Check sheet for the modelled part. Datum: model origin and axes. Units: mm. A direction names the side the tool comes from. Round coordinates to 2 decimals unless told otherwise and drop trailing zeros. Order: outer loops, then holes, each group sorted by start corner. A loop starts at its lowest first (then second) coordinate and runs counter-clockwise, first axis right, second up. Notation, with made-up numbers: (19.25, -35.75) -> (78.25, -35.75) arc R5 cw to (78.25, -31.75) -> close; hole circle Ø10 at (1.25, 87). An arc over 180 degrees is marked (long way). Answer in a Markdown table with one row per item. Add a question column.
1. Depth check by flat-ended pin: P1, Ø1, axis at y = 14, z = 1, coming from the +X side; P2, Ø0.5, axis at x = -56, z = 2, coming from the +Y side; P3, Ø0.6, axis at y = 13.5, z = 1.5, coming from the -X side. Enter the tip coordinate at first touch or a pass-through.
2. Sectioned sample at C-C, the plane x = 51. Record the boundary of the cut face in (y, z), then the cut area to 3 significant figures.
3. Material ranges on L1, parallel to Y at x = 9, z = 1.55; L2, parallel to X at y = 10.5, z = 0.35; L3, parallel to X at y = 9, z = 1.85, recorded low to high. Write a range as from..to.
4. Access from +Z, -Z, +X, -X, +Y, -Y to the whole of each face (thin tool, end or side, straight path). Record for faces 1 (the flat face through (1, 0, 0)), 2 (the flat face through (-55.525, -5, 2)).
5. Draft check along X on faces 3 (the cylindrical face through (4.18, 5.45, 1.52)), 4 (the flat face through (1, 0, 3)), 5 (the cylindrical face through (55.273, 12.743, 1.479)). Enter one of: +X half, -X half, draft (parallel to the pull), parting line (faces both ways), or undercut.
6. Sectioned sample at B-B, the plane y = -2.25. Record the boundary of the cut face in (x, z) (3 decimals), then the cut area to 3 significant figures.
7. Sectioned sample at A-A, the plane z = 1.2. Record the boundary of the cut face in (x, y) (3 decimals).
8. Sectioned sample at D-D, the plane y = 12. Record the boundary of the cut face in (x, z), then the cut area to 3 significant figures.
```python
from build123d import *

# Parameters (mm, degrees)
SKETCH1_R           = 3.8
BOSS_EXTRUDE2_DEPTH = 3
SKETCH2_R           = 4.4
BOSS_EXTRUDE3_DEPTH = 25
CUT_EXTRUDE3_START  = -1
SKETCH10_R          = 4.4
CUT_EXTRUDE3_DEPTH  = 1
CUT_EXTRUDE4_DEPTH  = 50
SKETCH12_R          = 4.55
CUT_EXTRUDE6_DEPTH  = 50
CUT_EXTRUDE7_DEPTH  = 25


with BuildPart() as part:
    # Sketch1 → Boss-Extrude2 (new body)
    with BuildSketch(Plane.XY):
        with BuildLine():
            Line((-48.125, 15.75), (48.125, 15.75))
            ThreePointArc((48.125, 15.75), (55.196067812, 12.821067812), (58.125, 5.75))
            Line((58.125, 5.75), (58.125, -15.75))
            Line((58.125, -15.75), (-58.125, -15.75))
            Line((-58.125, -15.75), (-58.125, 5.75))
            ThreePointArc((-58.125, 5.75), (-55.196067812, 12.821067812), (-48.125, 15.75))
        make_face()
        with Locations((31.875, -2.25)):
            Circle(SKETCH1_R, mode=Mode.SUBTRACT)
        with Locations((-31.875, 0.25)):
            Circle(SKETCH1_R, mode=Mode.SUBTRACT)
    extrude(amount=BOSS_EXTRUDE2_DEPTH)

    # Sketch2 → Boss-Extrude3 (add)
    with BuildSketch(Plane.XY.offset(3)):
        with Locations((8.725, 5.25)):
            Circle(SKETCH2_R)
        with Locations((-10.185, -4.75)):
            Circle(SKETCH2_R)
        with BuildLine():
            Line((55.625, 5.75), (55.625, -15.75))
            Line((55.625, -15.75), (58.125, -15.75))
            Line((58.125, -15.75), (58.125, 5.25))
            Line((58.125, 5.25), (58.125, 5.75))
            ThreePointArc((58.125, 5.75), (55.196067812, 12.821067812), (48.125, 15.75))
            Line((48.125, 15.75), (48.125, 13.25))
            ThreePointArc((48.125, 13.25), (53.428300859, 11.053300859), (55.625, 5.75))
        make_face()
        with BuildLine():
            Line((-58.125, -15.75), (-55.625, -15.75))
            Line((-55.625, -15.75), (-55.625, 5.75))
            ThreePointArc((-55.625, 5.75), (-53.428300859, 11.053300859), (-48.125, 13.25))
            Line((-48.125, 13.25), (-48.125, 15.75))
            ThreePointArc((-48.125, 15.75), (-55.196067812, 12.821067812), (-58.125, 5.75))
            Line((-58.125, 5.75), (-58.125, 5.25))
            Line((-58.125, 5.25), (-58.125, -15.75))
        make_face()
    extrude(amount=BOSS_EXTRUDE3_DEPTH)

    # Sketch10 → Cut-Extrude3 (cut)
    with BuildSketch(Plane.XY.offset(28).offset(CUT_EXTRUDE3_START)):
        with Locations((8.725, 5.25)):
            Circle(SKETCH10_R)
        with Locations((-10.185, -4.75)):
            Circle(SKETCH10_R)
    extrude(amount=CUT_EXTRUDE3_DEPTH, mode=Mode.SUBTRACT)

    # Sketch5 → Cut-Extrude4 (cut)
    with BuildSketch(Plane.XY.offset(28)):
        with BuildLine():
            Line((55.525, -14.7), (55.525, 5.75))
            ThreePointArc((55.525, 5.75), (53.322114584, 11.017826876), (48.025, 13.149324293))
            Line((48.025, 13.149324293), (48.025, 14.384631142))
            ThreePointArc((48.025, 14.384631142), (54.933874825, 11.243952477), (56.946937757, 3.926576481))
            Line((56.946937757, 3.926576481), (57.075693637, -14.7))
            Line((57.075693637, -14.7), (55.525, -14.7))
        make_face()
        with BuildLine():
            Line((-56.946937757, 3.926576481), (-57.075693637, -14.7))
            Line((-57.075693637, -14.7), (-55.525, -14.7))
            Line((-55.525, -14.7), (-55.525, 5.75))
            ThreePointArc((-55.525, 5.75), (-53.322114584, 11.017826876), (-48.025, 13.149324293))
            Line((-48.025, 13.149324293), (-48.025, 14.384631142))
            ThreePointArc((-48.025, 14.384631142), (-54.933874825, 11.243952477), (-56.946937757, 3.926576481))
        make_face()
    extrude(amount=-CUT_EXTRUDE4_DEPTH, mode=Mode.SUBTRACT)

    # Sketch12 → Cut-Extrude6 (cut)
    with BuildSketch(Plane.XY.offset(27)):
        with Locations((-10.185, -4.75)):
            Circle(SKETCH12_R)
        with Locations((8.725, 5.25)):
            Circle(SKETCH12_R)
    extrude(amount=-CUT_EXTRUDE6_DEPTH, mode=Mode.SUBTRACT)

    # Sketch13 → Cut-Extrude7 (cut)
    with BuildSketch(Plane.XY.offset(28)):
        with BuildLine():
            Line((57.075693637, -14.7), (55.625, -14.7))
            Line((55.625, -14.7), (55.625, -15.75))
            Line((55.625, -15.75), (58.125, -15.75))
            Line((58.125, -15.75), (58.125, 5.75))
            ThreePointArc((58.125, 5.75), (55.196067812, 12.821067812), (48.125, 15.75))
            Line((48.125, 15.75), (48.125, 14.385189819))
            ThreePointArc((48.125, 14.385189819), (54.966220263, 11.205822827), (56.946937757, 3.926576481))
            Line((56.946937757, 3.926576481), (57.075693637, -14.7))
        make_face()
        with BuildLine():
            Line((-48.125, 14.385189819), (-48.125, 15.75))
            ThreePointArc((-48.125, 15.75), (-55.196067812, 12.821067812), (-58.125, 5.75))
            Line((-58.125, 5.75), (-58.125, -15.75))
            Line((-58.125, -15.75), (-55.625, -15.75))
            Line((-55.625, -15.75), (-55.625, -14.7))
            Line((-55.625, -14.7), (-57.075693637, -14.7))
            Line((-57.075693637, -14.7), (-56.946937757, 3.926576481))
            ThreePointArc((-56.946937757, 3.926576481), (-54.966220263, 11.205822827), (-48.125, 14.385189819))
        make_face()
    extrude(amount=-CUT_EXTRUDE7_DEPTH, mode=Mode.SUBTRACT)


solid = part.part
```
Answer key:
| question | item | result |
|---|---|---|
| 1 | P1 | stops at x = 54.44 |
| 1 | P2 | stops at y = 12.22 |
| 1 | P3 | stops at x = -54.8 |
| 2 | outline | (-15.75, 0) -> (12.57, 0) -> (12.57, 3) -> (-15.75, 3) -> close; (13.91, 0) -> (15.33, 0) -> (15.33, 3) -> (13.91, 3) -> close |
| 2 | area | 89.2 mm² |
| 3 | L1 | y = -15.75..0.71, 9.79..15.75 |
| 3 | L2 | x = -56.92..-55.5, -53.8..53.8, 55.5..56.92 |
| 3 | L3 | x = -57.58..-56.33, -54.77..6.15, 11.3..54.77, 56.33..57.58 |
| 4 | face 1 | -Z, +X, -X, +Y, -Y |
| 4 | face 2 | +Z, -Z |
| 5 | face 3 | undercut |
| 5 | face 4 | draft |
| 5 | face 5 | +X half |
| 6 | outline | (-58.125, 0) -> (-56.99, 0) -> (-56.99, 3) -> (-58.125, 3) -> close; (-55.525, 0) -> (-34.737, 0) -> (-34.737, 3) -> (-55.525, 3) -> close; (-29.013, 0) -> (-13.987, 0) -> (-13.987, 3) -> (-29.013, 3) -> close; (-6.383, 0) -> (28.075, 0) -> (28.075, 3) -> (-6.383, 3) -> close; (35.675, 0) -> (55.525, 0) -> (55.525, 3) -> (35.675, 3) -> close; (56.99, 0) -> (58.125, 0) -> (58.125, 3) -> (56.99, 3) -> close |
| 6 | area | 277 mm² |
| 7 | outline | (-58.125, -15.75) -> (58.125, -15.75) -> (58.125, 5.75) arc R10 ccw to (48.125, 15.75) -> (-48.125, 15.75) arc R10 ccw to (-58.125, 5.75) -> close; hole (-57.076, -14.7) -> (-55.525, -14.7) -> (-55.525, 5.75) arc R7.4 cw to (-48.025, 13.149) -> (-48.025, 14.385) arc R8.95 ccw to (-56.947, 3.927) -> close; hole circle Ø7.6 at (-31.875, 0.25); hole circle Ø9.1 at (-10.185, -4.75); hole circle Ø9.1 at (8.725, 5.25); hole circle Ø7.6 at (31.875, -2.25); hole (48.025, 13.149) arc R7.4 cw to (55.525, 5.75) -> (55.525, -14.7) -> (57.076, -14.7) -> (56.947, 3.927) arc R8.95 ccw to (48.025, 14.385) -> close |
| 8 | outline | (-55.93, 0) -> (-54.21, 0) -> (-54.21, 3) -> (-55.93, 3) -> close; (-52.09, 0) -> (52.09, 0) -> (52.09, 3) -> (-52.09, 3) -> close; (54.21, 0) -> (55.93, 0) -> (55.93, 3) -> (54.21, 3) -> close |
| 8 | area | 323 mm² |
